Check sheet for the drawn part. Datum: minimum x, y, z corner. Units: mm. A direction names the side the tool comes from. Give positions to 0.01 mm unless a question says otherwise; leave off trailing zeros. Order: outer loops, then holes, each group sorted by start corner. A loop starts at its lowest first (then second) coordinate and runs counter-clockwise, first axis right, second up. Notation, with made-up numbers: (59.25, 66.5) -> (93.25, 66.5) arc R24 cw to (93.25, 88.5) -> close; hole circle Ø5 at (28, 72.5). An arc over 180 degrees is marked (long way). Answer in a Markdown table with one row per item. Add a question column.
(1) Set-up check for the marked faces 1, 2, 3 and 4: record each of +Z, -Z, +X, -X, +Y, -Y from which the full face is reachable in a straight line by a thin tool's end or side.
(2) Cross-section at B-B (y = 27). Record the cut outline in (x, z), then the cut area to 3 significant figures.
(3) Cross-section at A-A (x = 10). Record the cut outline in (y, z), then the cut area to 3 significant figures.
(4) Cross-section at D-D (x = 5). Record the cut outline in (y, z), then the cut area to 3 significant figures.
(5) Cross-section at C-C (z = 8). Record the cut outline in (x, y), then the cut area to 3 significant figures.
(6) Thickness scan on L1, parallel to Y at x = 0.7, z = 8; L2, parallel to Y at x = 4.5, z = 5; L3, parallel to Z at x = 10, y = 8.95. Record the ranges inside material, lowest first. Write a range as [from, to].
(7) Release check for a two-part mould opening along Z. For the marked faces 5, 6, 7 and 8 record: released by +Z, released by -Z, zero draft, split by the parting line, or undercut.
(8) Go/stop test with flat-tipped pins: pin 1 (3.5 mm diameter, centred on x = 10.5, z = 6, fed in from +Y); pin 2 (7.5 mm diameter, centred on y = 2, z = 11.5, fed in from +X); pin 3 (3.5 mm diameter, centred on x = 7.5, z = 8.5, fed in from -Y); pin 4 (2.5 mm diameter, centred on y = 27, z = 8, fed in from -X). Record where each tip stops, or that it passes through.
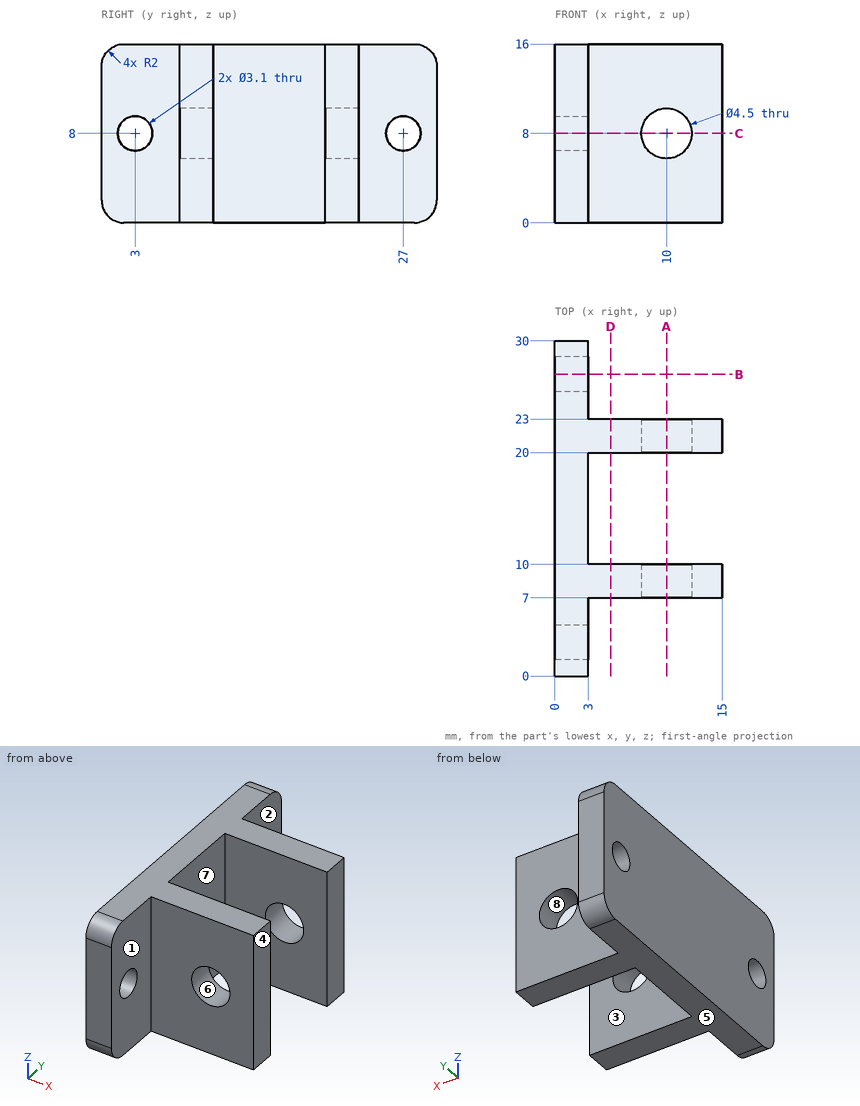
Answer below:
| question | item | result |
|---|---|---|
| 1 | face 1 | +Z, -Z, +X, -Y |
| 1 | face 2 | +Z, -Z, +X, +Y |
| 1 | face 3 | +Z, -Z, +X |
| 1 | face 4 | +Z, -Z, +X, +Y, -Y |
| 2 | outline | (0, 0) -> (3, 0) -> (3, 6.45) -> (0, 6.45) -> close; (0, 9.55) -> (3, 9.55) -> (3, 16) -> (0, 16) -> close |
| 2 | area | 38.7 mm² |
| 3 | outline | (7, 0) -> (10, 0) -> (10, 5.75) -> (7, 5.75) -> close; (7, 10.25) -> (10, 10.25) -> (10, 16) -> (7, 16) -> close; (20, 0) -> (23, 0) -> (23, 5.75) -> (20, 5.75) -> close; (20, 10.25) -> (23, 10.25) -> (23, 16) -> (20, 16) -> close |
| 3 | area | 69.0 mm² |
| 4 | outline | (7, 0) -> (10, 0) -> (10, 16) -> (7, 16) -> close; (20, 0) -> (23, 0) -> (23, 16) -> (20, 16) -> close |
| 4 | area | 96.0 mm² |
| 5 | outline | (0, 0) -> (3, 0) -> (3, 1.45) -> (0, 1.45) -> close; (0, 4.55) -> (3, 4.55) -> (3, 7) -> (7.75, 7) -> (7.75, 10) -> (3, 10) -> (3, 20) -> (7.75, 20) -> (7.75, 23) -> (3, 23) -> (3, 25.45) -> (0, 25.45) -> close; (0, 28.55) -> (3, 28.55) -> (3, 30) -> (0, 30) -> close; (12.25, 7) -> (15, 7) -> (15, 10) -> (12.25, 10) -> close; (12.25, 20) -> (15, 20) -> (15, 23) -> (12.25, 23) -> close |
| 5 | area | 116 mm² |
| 6 | L1 | y = [0, 1.45], [4.55, 25.45], [28.55, 30] |
| 6 | L2 | y = [7, 10], [20, 23] |
| 6 | L3 | z = [0, 5.75], [10.25, 16] |
| 7 | face 5 | released by -Z |
| 7 | face 6 | undercut |
| 7 | face 7 | zero draft |
| 7 | face 8 | undercut |
| 8 | pin 1 | stops at y = 23 |
| 8 | pin 2 | stops at x = 3 |
| 8 | pin 3 | stops at y = 7 |
| 8 | pin 4 | passes through |
